Build history of the part. All positions in model axes, mm. A direction names the side the tool comes from. Round coordinates to 2 decimals unless told otherwise and drop trailing zeros. Loops run counter-clockwise (first coordinate to the right, second up) from the corner with the lowest first, then second, coordinate; pieces in that order, holes last. Notation, with made-up numbers: (16.5, 45.25) - (65.5, 45.25) arc R21 cw to (65.5, 84.25) - close; hole circle Ø1 at (80, 46). An arc over 180 degrees is marked (long way). Use a Markdown table: item, result.
from build123d import *

# Parameters (mm, degrees)
IZIM1_R                     = 25
Y_KSEKLIK_EKSTR_ZYON1_DEPTH = 5
IZIM2_R                     = 33
Y_KSEKLIK_EKSTR_ZYON2_DEPTH = 33


with BuildPart() as part:
    # Çizim1 → Yükseklik-Ekstrüzyon1 (new body, symmetric)
    with BuildSketch(Plane.XY):
        Circle(IZIM1_R)
        with BuildLine():
            Line((-5, 16.248076809), (-4.411764706, 14.336538361))
            ThreePointArc((-4.411764706, 14.336538361), (0, 15), (4.411764706, 14.336538361))
            Line((4.411764706, 14.336538361), (5, 16.248076809))
            ThreePointArc((5, 16.248076809), (8.5, 14.722431864), (11.571247279, 12.454165424))
            Line((11.571247279, 12.454165424), (10.20992407, 10.988969491))
            ThreePointArc((10.20992407, 10.988969491), (12.990381057, 7.5), (14.621688776, 3.34756887))
            Line((14.621688776, 3.34756887), (16.571247279, 3.793911386))
            ThreePointArc((16.571247279, 3.793911386), (17, 0), (16.571247279, -3.793911386))
            Line((16.571247279, -3.793911386), (14.621688776, -3.34756887))
            ThreePointArc((14.621688776, -3.34756887), (12.990381057, -7.5), (10.20992407, -10.988969491))
            Line((10.20992407, -10.988969491), (11.571247279, -12.454165424))
            ThreePointArc((11.571247279, -12.454165424), (8.5, -14.722431864), (5, -16.248076809))
            Line((5, -16.248076809), (4.411764706, -14.336538361))
            ThreePointArc((4.411764706, -14.336538361), (0, -15), (-4.411764706, -14.336538361))
            Line((-4.411764706, -14.336538361), (-5, -16.248076809))
            ThreePointArc((-5, -16.248076809), (-8.5, -14.722431864), (-11.571247279, -12.454165424))
            Line((-11.571247279, -12.454165424), (-10.20992407, -10.988969491))
            ThreePointArc((-10.20992407, -10.988969491), (-12.990381057, -7.5), (-14.621688776, -3.34756887))
            Line((-14.621688776, -3.34756887), (-16.571247279, -3.793911386))
            ThreePointArc((-16.571247279, -3.793911386), (-17, 0), (-16.571247279, 3.793911386))
            Line((-16.571247279, 3.793911386), (-14.621688776, 3.34756887))
            ThreePointArc((-14.621688776, 3.34756887), (-12.990381057, 7.5), (-10.20992407, 10.988969491))
            Line((-10.20992407, 10.988969491), (-11.571247279, 12.454165424))
            ThreePointArc((-11.571247279, 12.454165424), (-8.5, 14.722431864), (-5, 16.248076809))
        make_face(mode=Mode.SUBTRACT)
    extrude(amount=Y_KSEKLIK_EKSTR_ZYON1_DEPTH, both=True)

    # Çizim2 → Yükseklik-Ekstrüzyon2 (add)
    with BuildSketch(Plane(origin=(0, 0, -5), x_dir=(-1, 0, 0), z_dir=(0, 0, -1))):
        Circle(IZIM2_R)
        with BuildLine():
            Line((-5, 16.248076809), (-4.411764706, 14.336538361))
            ThreePointArc((-4.411764706, 14.336538361), (0, 15), (4.411764706, 14.336538361))
            Line((4.411764706, 14.336538361), (5, 16.248076809))
            ThreePointArc((5, 16.248076809), (8.5, 14.722431864), (11.571247279, 12.454165424))
            Line((11.571247279, 12.454165424), (10.20992407, 10.988969491))
            ThreePointArc((10.20992407, 10.988969491), (12.990381057, 7.5), (14.621688776, 3.34756887))
            Line((14.621688776, 3.34756887), (16.571247279, 3.793911386))
            ThreePointArc((16.571247279, 3.793911386), (17, 0), (16.571247279, -3.793911386))
            Line((16.571247279, -3.793911386), (14.621688776, -3.34756887))
            ThreePointArc((14.621688776, -3.34756887), (12.990381057, -7.5), (10.20992407, -10.988969491))
            Line((10.20992407, -10.988969491), (11.571247279, -12.454165424))
            ThreePointArc((11.571247279, -12.454165424), (8.5, -14.722431864), (5, -16.248076809))
            Line((5, -16.248076809), (4.411764706, -14.336538361))
            ThreePointArc((4.411764706, -14.336538361), (0, -15), (-4.411764706, -14.336538361))
            Line((-4.411764706, -14.336538361), (-5, -16.248076809))
            ThreePointArc((-5, -16.248076809), (-8.5, -14.722431864), (-11.571247279, -12.454165424))
            Line((-11.571247279, -12.454165424), (-10.20992407, -10.988969491))
            ThreePointArc((-10.20992407, -10.988969491), (-12.990381057, -7.5), (-14.621688776, -3.34756887))
            Line((-14.621688776, -3.34756887), (-16.571247279, -3.793911386))
            ThreePointArc((-16.571247279, -3.793911386), (-17, 0), (-16.571247279, 3.793911386))
            Line((-16.571247279, 3.793911386), (-14.621688776, 3.34756887))
            ThreePointArc((-14.621688776, 3.34756887), (-12.990381057, 7.5), (-10.20992407, 10.988969491))
            Line((-10.20992407, 10.988969491), (-11.571247279, 12.454165424))
            ThreePointArc((-11.571247279, 12.454165424), (-8.5, 14.722431864), (-5, 16.248076809))
        make_face(mode=Mode.SUBTRACT)
    extrude(amount=Y_KSEKLIK_EKSTR_ZYON2_DEPTH)


solid = part.part
Q1. Cut at A-A, the plane x = 0. List the corners of the cut face in (y, z).
Results found:
| item | result |
|---|---|
| outline | (-33, -38) - (-15, -38) - (-15, 5) - (-25, 5) - (-25, -5) - (-33, -5) - close; (15, -38) - (33, -38) - (33, -5) - (25, -5) - (25, 5) - (15, 5) - close |
Q2. Cut at C-C, the plane z = -17.5. List the corners of the cut face in (x, y).
Results found:
| item | result |
|---|---|
| outline | circle Ø66 at (0, 0); hole (-16.57, -3.79) - (-14.62, -3.35) arc R15 ccw to (-10.21, -10.99) - (-11.57, -12.45) arc R17 ccw to (-5, -16.25) - (-4.41, -14.34) arc R15 ccw to (4.41, -14.34) - (5, -16.25) arc R17 ccw to (11.57, -12.45) - (10.21, -10.99) arc R15 ccw to (14.62, -3.35) - (16.57, -3.79) arc R17 ccw to (16.57, 3.79) - (14.62, 3.35) arc R15 ccw to (10.21, 10.99) - (11.57, 12.45) arc R17 ccw to (5, 16.25) - (4.41, 14.34) arc R15 ccw to (-4.41, 14.34) - (-5, 16.25) arc R17 ccw to (-11.57, 12.45) - (-10.21, 10.99) arc R15 ccw to (-14.62, 3.35) - (-16.57, 3.79) arc R17 ccw to start |
Q3. Which spindle directions (+Z, -Z, +X, -X, +Y, -Y) get a long thin tool onto all of the face, cutting with end or side? Do faces 4 (the face through (23.846, 7.509, 0.07)), 5 (the face through (15.61, 3.574, -16.199)), 6 (the face through (-14, -7, -38)). Say none if no direction does.
Results found:
| item | result |
|---|---|
| face 4 | +Z |
| face 5 | +Z, -Z |
| face 6 | -Z, +X, -X, +Y, -Y |
Q4. Probe line 1 (Z direction, x = 1, y = 30); line 2 (X direction, y = 12.5, z = -31); line 3 (X direction, y = 9.5, z = -7.5). List the from-to ranges inside material, lowest first.
Results found:
| item | result |
|---|---|
| line 1 | z = -38 to -5 |
| line 2 | x = -30.54 to -11.52, 11.52 to 30.54 |
| line 3 | x = -31.6 to -11.61, 11.61 to 31.6 |
Q5. Cut at D-D, the plane y = -24. List the corners of the cut face in (x, z).
Results found:
| item | result |
|---|---|
| outline | (-22.65, -38) - (22.65, -38) - (22.65, -5) - (7, -5) - (7, 5) - (-7, 5) - (-7, -5) - (-22.65, -5) - close |
Q6. Cut at B-B, the plane y = 0. List the corners of the cut face in (x, z), plus the area to 3 significant figures.
Results found:
| item | result |
|---|---|
| outline | (-33, -38) - (-17, -38) - (-17, 5) - (-25, 5) - (-25, -5) - (-33, -5) - close; (17, -38) - (33, -38) - (33, -5) - (25, -5) - (25, 5) - (17, 5) - close |
| area | 1,220 mm2 |
Q7. Drop flat-ended pins along their axis: pin 1 (6 mm diameter, centred on y = -9.5, z = -23, fed in from +X); pin 2 (1.5 mm diameter, centred on x = -16, y = -22.5, fed in from +Z); pin 3 (3 mm diameter, centred on x = 11, z = -1.5, fed in from +Y). Give the stop position or say it passes through.
Results found:
| item | result |
|---|---|
| pin 1 | stops at x = 32.35 |
| pin 2 | stops at z = -5 |
| pin 3 | stops at y = 23.12 |
Q8. Pull direction Y, two halves, no side cores. Call faces 1 (the face through (-30.5, -12.6, -21.3)), 2 (the face through (11, -11, 5)), 3 (the face through (0, 15, -16)): pulls with the +Y half, pulls with the -Y half, needs draft (parallel to the pull), parting line crosses it, or undercut.
Results found:
| item | result |
|---|---|
| face 1 | parting line crosses it |
| face 2 | needs draft |
| face 3 | undercut |
